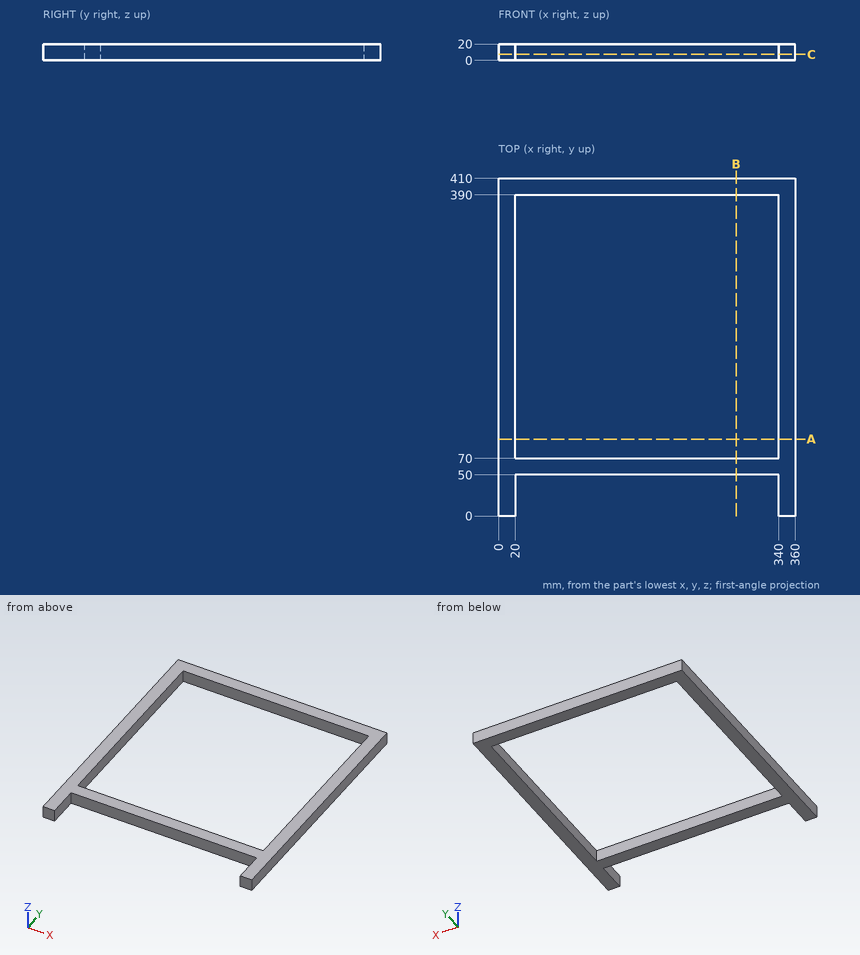
Source: three-view drawing plus pictorial views. Frame: mm from the lowest corner of the part. Round coordinates to 2 decimals unless told otherwise and drop trailing zeros. Order: outer loops, then holes, each group sorted by start corner. A loop starts at its lowest first (then second) coordinate and runs counter-clockwise, first axis right, second up. Notation, with made-up numbers: (-32, 42.25) -> (-5, 42.25) arc R26 cw to (-5, 67.25) -> close; hole circle Ø6 at (53, -29.5). An arc over 180 degrees is marked (long way). Use one line per item in the form item = value.
(1) Section A-A on y = 93.5. Return loops of the section in (x, z).
Results list:
outline = (0, 0) -> (20, 0) -> (20, 20) -> (0, 20) -> close; (340, 0) -> (360, 0) -> (360, 20) -> (340, 20) -> close
(2) Section B-B on x = 288.5. Return loops of the section in (y, z), and give its area (3 significant figures).
Results list:
outline = (50, 0) -> (70, 0) -> (70, 20) -> (50, 20) -> close; (390, 0) -> (410, 0) -> (410, 20) -> (390, 20) -> close
area = 800 mm^2
(3) Ray query, probe 1 along X at (y, z) = (256.5, 2.5); probe 2 along Y at (x, z) = (213, 14). Return the intervals inside material, ascending. Write a range as [from, to].
Results list:
probe_1 = [0, 20], [340, 360]
probe_2 = [50, 70], [390, 410]
(4) First-contact query: pin 1 Ø6 at (x, z) = (98, 10) entering from -Y; pin 2 Ø5 at (y, z) = (255, 6.5) entering from -X. Flat tips, straight axial feed; report the tip coordinate or a pass-through.
Results list:
pin_1 = 50
pin_2 = 0
(5) Section C-C on z = 7.25. Return loops of the section in (x, y), and give its area (3 significant figures).
Results list:
outline = (0, 0) -> (20, 0) -> (20, 50) -> (340, 50) -> (340, 0) -> (360, 0) -> (360, 410) -> (0, 410) -> close; hole (20, 70) -> (340, 70) -> (340, 390) -> (20, 390) -> close
area = 29,200 mm^2
